Autodesk Inventor part; units mm, degrees
ref_plane "YZ Plane" through (0, 0, 0) normal (1, 0, 0) x (0, 1, 0)
ref_plane "XZ Plane" through (0, 0, 0) normal (0, 1, 0) x (-1, 0, 0)
ref_plane "XY Plane" through (0, 0, 0) normal (0, 0, 1) x (1, 0, 0)
sketch "Sketch1" plane through (0, 0, 0) normal (0, 0, 1) x (1, 0, 0)
  line L0 (-28.2, 28.2) -> (28.2, 28.2)
  line L1 (28.2, 28.2) -> (28.2, -28.2)
  line L2 (28.2, -28.2) -> (-28.2, -28.2)
  line L3 (-28.2, -28.2) -> (-28.2, 28.2)
  line L4 (-28.2, 28.2) -> (28.2, -28.2) construction
  line L5 (28.2, 28.2) -> (-28.2, -28.2) construction
  circle A0 centre (25.45, 16.4) radius 1.5
  circle A1 centre (25.45, -16.4) radius 1.5
  line L6 (0, 0) -> (0, 28.2) construction
  circle A2 centre (-25.45, 16.4) radius 1.5
  circle A3 centre (-25.45, -16.4) radius 1.5
  circle A4 centre (23.55, 23.55) radius 3.1
  circle A5 centre (-23.55, 23.55) radius 3.1
  circle A6 centre (-23.55, -23.55) radius 3.1
  circle A7 centre (23.55, -23.55) radius 3.1
  circle A8 centre (0, 0) radius 20
  line L7 (-28.2, 28.2) -> (13.2, 28.2)
  line L8 (13.2, 28.2) -> (13.2, 38.2)
  line L9 (13.2, 38.2) -> (-28.2, 38.2)
  line L10 (-28.2, 38.2) -> (-28.2, 28.2)
  circle A9 centre (-23.2, 33.2) radius 1.5
  circle A10 centre (8.2, 33.2) radius 1.5
  line L11 (13.2, -28.2) -> (-28.2, -28.2)
  line L12 (-28.2, -28.2) -> (-28.2, -44.2)
  line L13 (-28.2, -44.2) -> (13.2, -44.2)
  line L14 (13.2, -44.2) -> (13.2, -28.2)
  circle A11 centre (-23.2, -39.2) radius 1.5
  circle A12 centre (8.2, -39.2) radius 1.5
  line L15 (28.2, -28.2) -> (13.2, -28.2)
  line L16 (13.2, -28.2) -> (13.2, -34.2)
  line L17 (13.2, -34.2) -> (28.2, -34.2)
  line L18 (28.2, -34.2) -> (28.2, -28.2)
  point P0 (-28.2, -28.2)
  dimension "d0" = 3
  dimension "d1" = 56.4
  dimension "d2" = 16.4
  dimension "d3" = 25.45
  dimension "d4" = 56.4
  dimension "d5" = 3
  dimension "d6" = 16.4
  dimension "d7" = 25.45
  dimension "d8" = 6.2
  dimension "d9" = 23.55
  dimension "d10" = 23.55
  dimension "d13" = 360
  dimension "d17" = 40
  dimension "d18" = 10
  dimension "d19" = 15
  dimension "d20" = 3
  dimension "d21" = 3
  dimension "d22" = 5
  dimension "d23" = 5
  dimension "d24" = 5
  dimension "d25" = 5
  dimension "d26" = 16
  dimension "d27" = 15
  dimension "d28" = 0
  dimension "d29" = 3
  dimension "d30" = 3
  dimension "d31" = 5
  dimension "d32" = 5
  dimension "d33" = 5
  dimension "d34" = 5
  dimension "d35" = 6
extrude "Extrusion1" add sketch "Sketch1" along normal blind 4
sketch "Sketch3" plane through (0, 0, 4) normal (0, 0, 1) x (1, 0, 0)
  line L0 (28.2, -34.2) -> (28.2, 28.2)
  line L1 (28.2, 28.2) -> (13.2, 28.2)
  line L2 (13.2, 28.2) -> (13.2, 38.2)
  line L3 (13.2, 38.2) -> (-28.2, 38.2)
  line L4 (-28.2, 38.2) -> (-28.2, -44.2)
  line L5 (-28.2, -44.2) -> (13.2, -44.2)
  line L6 (13.2, -44.2) -> (13.2, -34.2)
  line L7 (13.2, -34.2) -> (28.2, -34.2)
  circle A0 centre (0, 0) radius 20
  circle A1 centre (25.45, 16.4) radius 1.5
  circle A2 centre (25.45, -16.4) radius 1.5
  circle A3 centre (-25.45, 16.4) radius 1.5
  circle A4 centre (-25.45, -16.4) radius 1.5
  circle A5 centre (23.55, 23.55) radius 3.1
  circle A6 centre (-23.55, 23.55) radius 3.1
  circle A7 centre (-23.55, -23.55) radius 3.1
  circle A8 centre (23.55, -23.55) radius 3.1
  circle A9 centre (-23.2, 33.2) radius 1.5
  circle A10 centre (8.2, 33.2) radius 1.5
  circle A11 centre (-23.2, -39.2) radius 1.5
  circle A12 centre (8.2, -39.2) radius 1.5
equation "\"d4\" = d1"
equation "\"d6\" = d2"
equation "\"d7\" = d3"
properties part number "MotorHolder_3D" material "Aluminum 6061, Welded"
The listing builds one solid part. Answer for the finished solid, in the listing's coordinates (mm). A direction names the side the tool comes from. Coordinates: 2 decimals unless noted, no trailing zeros. Write each loop counter-clockwise with the first axis right and the second up, starting at its lowest first coordinate (ties: lowest second). Pieces come first, ordered by that corner, then holes. Notation, with made-up numbers: (44.5, 40) - (101.5, 40) arc R16 cw to (101.5, 66) - close; hole circle Ø9 at (-24.75, 16). An arc over 180 degrees is marked (long way). Return JSON: item names as keys, results as strings. Group by question number.
Q1. The part is cut by section B-B on z = 2.55. State how many separate pieces and enclosed holes the cut face has, and give its area (3 significant figures).
Q2. Find the intervals of material crossed by line 1 along Y through (x, z) = (23.55, 2.45); line 2 along Y through (x, z) = (-23.55, 2.35); line 3 along Y through (x, z) = (-25.45, 2.75), in increasing order. Write a range as [from, to].
Q3. For a pull along Y with two mould halves and no side action, classify faces 4 (the flat face through (-8, -44.2, 2)), 5 (the cylindrical face through (23.95, 16.33, 1.97)), 6 (the flat face through (21, 28.2, 2)) as +Y half, -Y half, draft (parallel to the pull), parting line (faces both ways), or undercut.
Q4. The part is cut by section C-C on y = 7. Write down the section's boundary in (x, z) (3 decimals).
Q5. The part is cut by section A-A on y = -23.55. Write down the section's boundary in (x, z).
Q6. Which of the six approach directions +Z, -Z, +X, -X, +Y, -Y give full straight-line access (tool end or side, diameter ignored) to faces 1 (the flat face through (13.2, -39, 2)), 2 (the flat face through (13.2, 33, 2)), 3 (the cylindrical face through (-23.395, 31.713, 1.972))?
Q7. Flat-ended cylindrical pins translate along their axes: pin 1 Ø1.8 at (x, y) = (8.2, -39.2) entering from +Z; pin 2 Ø2 at (x, z) = (21.5, 2.5) entering from -Y; pin 3 Ø1.2 at (y, z) = (-39, 2.5) entering from +X. Find the tip coordinate at first contact, or state that the pin passes through.
Q8. The part is cut by section D-D on x = -13.5. Write down the section's boundary in (y, z).
Evaluation:
{
 "1": {"separate pieces": "1", "enclosed holes": "13", "area": "2,910 mm2"},
 "2": {"line 1": "y = [-34.2, -26.65], [-20.45, 20.45], [26.65, 28.2]", "line 2": "y = [-44.2, -40.66], [-37.74, -26.65], [-20.45, 20.45], [26.65, 31.74], [34.66, 38.2]", "line 3": "y = [-44.2, -26], [-21.1, -17.9], [-14.9, 14.9], [17.9, 21.1], [26, 38.2]"},
 "3": {"face 4": "-Y half", "face 5": "undercut", "face 6": "+Y half"},
 "4": {"outline": "(-28.2, 0) - (-18.735, 0) - (-18.735, 4) - (-28.2, 4) - close; (18.735, 0) - (28.2, 0) - (28.2, 4) - (18.735, 4) - close"},
 "5": {"outline": "(-28.2, 0) - (-26.65, 0) - (-26.65, 4) - (-28.2, 4) - close; (-20.45, 0) - (20.45, 0) - (20.45, 4) - (-20.45, 4) - close; (26.65, 0) - (28.2, 0) - (28.2, 4) - (26.65, 4) - close"},
 "6": {"face 1": "+Z, -Z, +X, -Y", "face 2": "+Z, -Z, +X, +Y", "face 3": "+Z, -Z"},
 "7": {"pin 1": "passes through", "pin 2": "stops at y = -34.2", "pin 3": "stops at x = 13.2"},
 "8": {"outline": "(-44.2, 0) - (-14.76, 0) - (-14.76, 4) - (-44.2, 4) - close; (14.76, 0) - (38.2, 0) - (38.2, 4) - (14.76, 4) - close"}
}
